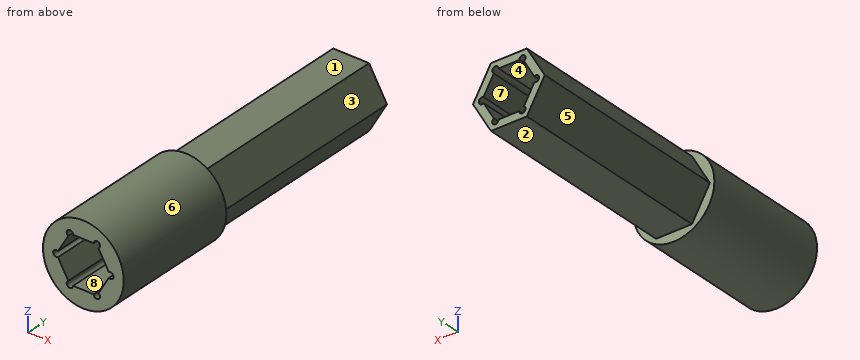
```python
from build123d import *

# Parameters (mm, degrees)
BOSS_EXTRUDE1_DEPTH     = 23
SKETCH2_R               = 4.45
BOSS_EXTRUDE2_DEPTH     = 14.3
CUT_EXTRUDE1_DEPTH      = 38.827172773
CUT_EXTRUDE1_DEPTH_BACK = 38.827172773
SKETCH4_R               = 0.35


with BuildPart() as part:
    # Sketch1 → Boss-Extrude1 (new body)
    with BuildSketch(Plane(origin=(0, 0, 0), x_dir=(1, 0, 0), z_dir=(0, 1, 0))):
        Polygon((1.977424672, 3.425), (-1.977424672, 3.425), (-3.954849344, 0), (-1.977424672, -3.425), (1.977424672, -3.425), (3.954849344, 0), align=None)
        Polygon((2.973353886, 0), (1.486676943, 2.575), (-1.486676943, 2.575), (-2.973353886, 0), (-1.486676943, -2.575), (1.486676943, -2.575), align=None, mode=Mode.SUBTRACT)
    extrude(amount=BOSS_EXTRUDE1_DEPTH)

    # Sketch2 → Boss-Extrude2 (add)
    with BuildSketch(Plane.XZ):
        with Locations(Location((0, 0, 0), (0, 0, 270))):
            Circle(SKETCH2_R)
        Polygon((2.973353886, 0), (1.486676943, 2.575), (-1.486676943, 2.575), (-2.973353886, 0), (-1.486676943, -2.575), (1.486676943, -2.575), align=None, mode=Mode.SUBTRACT)
    extrude(amount=BOSS_EXTRUDE2_DEPTH)

    # Sketch4 → Cut-Extrude1 (cut, two sides: drawn at the far end of the back side and taken through both)
    with BuildSketch(Plane(origin=(0, 23, 0), x_dir=(1, 0, 0), z_dir=(0, 1, 0)).offset(-CUT_EXTRUDE1_DEPTH_BACK)):
        with Locations((1.486676943, 2.575)):
            Circle(SKETCH4_R)
        with Locations((2.973353886, 0)):
            Circle(SKETCH4_R)
        with Locations((1.486676943, -2.575)):
            Circle(SKETCH4_R)
        with Locations((-1.486676943, -2.575)):
            Circle(SKETCH4_R)
        with Locations((-2.973353886, 0)):
            Circle(SKETCH4_R)
        with Locations((-1.486676943, 2.575)):
            Circle(SKETCH4_R)
    extrude(amount=CUT_EXTRUDE1_DEPTH + CUT_EXTRUDE1_DEPTH_BACK, mode=Mode.SUBTRACT)


solid = part.part
```
Check sheet for the modelled part. Datum: model origin and axes. Units: mm. Face numbers are marked on the shaded views. A direction names the side the tool comes from. Round coordinates to 2 decimals unless told otherwise and drop trailing zeros. Write each loop counter-clockwise with the first axis right and the second up, starting at its lowest first coordinate (ties: lowest second). Pieces come first, ordered by that corner, then holes. Notation, with made-up numbers: (54, -12) -> (62, -12) arc R22 cw to (62, 19) -> close; hole circle Ø6 at (-36, -6.5). An arc over 180 degrees is marked (long way). Put each result on its own line as item: value.
(1) Go/stop test with flat-tipped pins: pin 1 Ø3 at (y, z) = (8, 3) entering from -X; pin 2 Ø5 at (x, z) = (-1, -2) entering from +Y; pin 3 Ø1.5 at (x, z) = (0, -1.5) entering from -Y; pin 4 Ø0.7 at (x, y) = (-0.5, 3) entering from -Z (3 decimals). Record where each tip stops, or that it passes through.
Values found:
pin 1: stops at x = -3.09
pin 2: stops at y = 23
pin 3: passes through
pin 4: stops at z = -3.425
(2) Sectioned sample at B-B (y = -6). Enter the section's corners in (x, z) (3 decimals).
Values found:
outline: circle Ø8.9 at (0, 0); hole (-2.798, -0.303) -> (-1.662, -2.272) arc R0.35 ccw (long way) to (-1.137, -2.575) -> (1.137, -2.575) arc R0.35 ccw (long way) to (1.662, -2.272) -> (2.798, -0.303) arc R0.35 ccw (long way) to (2.798, 0.303) -> (1.662, 2.272) arc R0.35 ccw (long way) to (1.137, 2.575) -> (-1.137, 2.575) arc R0.35 ccw (long way) to (-1.662, 2.272) -> (-2.798, 0.303) arc R0.35 ccw (long way) to start
(3) Sectioned sample at A-A (x = 0). Enter the section's corners in (y, z) (3 decimals), plus the area to 3 significant figures.
Values found:
outline: (-14.3, -4.45) -> (0, -4.45) -> (0, -3.425) -> (23, -3.425) -> (23, -2.575) -> (-14.3, -2.575) -> close; (-14.3, 2.575) -> (23, 2.575) -> (23, 3.425) -> (0, 3.425) -> (0, 4.45) -> (-14.3, 4.45) -> close
area: 92.7 mm^2
(4) Tool access check on the marked faces 1, 2, 3 and 4. Record the directions out of +Z, -Z, +X, -X, +Y, -Y that give a thin tool (end or side, any length) a straight path to the whole face; none if there is none.
Values found:
face 1: +Z, +X, -X, +Y
face 2: -Z, +X, -X, +Y
face 3: +Z, +X, +Y
face 4: +Y, -Y
(5) Mould release check, pull along Z, two halves, no side actions. Record for the marked faces 5, 6, 7 and 8: released by +Z, released by -Z, zero draft, split by the parting line, or undercut.
Values found:
face 5: released by -Z
face 6: split by the parting line
face 7: undercut
face 8: undercut
(6) Sectioned sample at C-C (y = 17.5). Enter the section's corners in (x, z) (3 decimals), plus the area to 3 significant figures.
Values found:
outline: (-3.955, 0) -> (-1.977, -3.425) -> (1.977, -3.425) -> (3.955, 0) -> (1.977, 3.425) -> (-1.977, 3.425) -> close; hole (-2.798, -0.303) -> (-1.662, -2.272) arc R0.35 ccw (long way) to (-1.137, -2.575) -> (1.137, -2.575) arc R0.35 ccw (long way) to (1.662, -2.272) -> (2.798, -0.303) arc R0.35 ccw (long way) to (2.798, 0.303) -> (1.662, 2.272) arc R0.35 ccw (long way) to (1.137, 2.575) -> (-1.137, 2.575) arc R0.35 ccw (long way) to (-1.662, 2.272) -> (-2.798, 0.303) arc R0.35 ccw (long way) to start
area: 16.1 mm^2
(7) Material ranges on line 1 (Z direction, x = 0.75, y = 2) (3 decimals); line 2 (X direction, y = 5, z = -2.75); line 3 (Z direction, x = -1.5, y = 16) (3 decimals), recorded low to high.
Values found:
line 1: z = -3.425 to -2.575, 2.575 to 3.425
line 2: x = -2.37 to -1.79, -1.18 to 1.18, 1.79 to 2.37
line 3: z = -3.425 to -2.925, 2.925 to 3.425
